```python
from build123d import *

# Parameters (mm, degrees)
SKETCH1_W                    = 76.2
SKETCH1_H                    = 127
BOSS_EXTRUDE1_DEPTH          = 24.13
SKETCH2_R                    = 7.9375
F_1_2_13_THREADED_HOLE_DEPTH = 78.885280381
SKETCH3_R                    = 5.0419
F_3_8_THROUGH_HOLES_DEPTH    = 78.885280381
SKETCH4_R                    = 21.43125
CUT_EXTRUDE1_DEPTH           = 9.525


with BuildPart() as part:
    # Sketch1 → Boss-Extrude1 (new body)
    with BuildSketch(Plane(origin=(0, 0, 0), x_dir=(1, 0, 0), z_dir=(0, 1, 0))):
        Rectangle(SKETCH1_W, SKETCH1_H)
    extrude(amount=BOSS_EXTRUDE1_DEPTH)

    # Sketch2 → 1/2"-13 Threaded Hole (cut, through all)
    with BuildSketch(Plane(origin=(0, 24.13, 0), x_dir=(1, 0, 0), z_dir=(0, 1, 0))):
        with Locations(Location((0, 0, 0), (0, 0, 270))):
            Circle(SKETCH2_R)
    extrude(amount=-F_1_2_13_THREADED_HOLE_DEPTH, mode=Mode.SUBTRACT)

    # Sketch3 → 3/8" Through Holes (cut, through all)
    with BuildSketch(Plane(origin=(0, 24.13, 0), x_dir=(1, 0, 0), z_dir=(0, 1, 0))):
        with Locations(Location((-19.05, 44.45, 0), (0, 0, 270))):
            Circle(SKETCH3_R)
        with Locations(Location((19.05, 44.45, 0), (0, 0, 270))):
            Circle(SKETCH3_R)
        with Locations(Location((19.05, -44.45, 0), (0, 0, 270))):
            Circle(SKETCH3_R)
        with Locations(Location((-19.05, -44.45, 0), (0, 0, 270))):
            Circle(SKETCH3_R)
    extrude(amount=-F_3_8_THROUGH_HOLES_DEPTH, mode=Mode.SUBTRACT)

    # Sketch4 → Cut-Extrude1 (cut)
    with BuildSketch(Plane(origin=(0, 24.13, 0), x_dir=(1, 0, 0), z_dir=(0, 1, 0))):
        with Locations(Location((0, 0, 0), (0, 0, 270))):
            Circle(SKETCH4_R)
    extrude(amount=-CUT_EXTRUDE1_DEPTH, mode=Mode.SUBTRACT)


solid = part.part
```
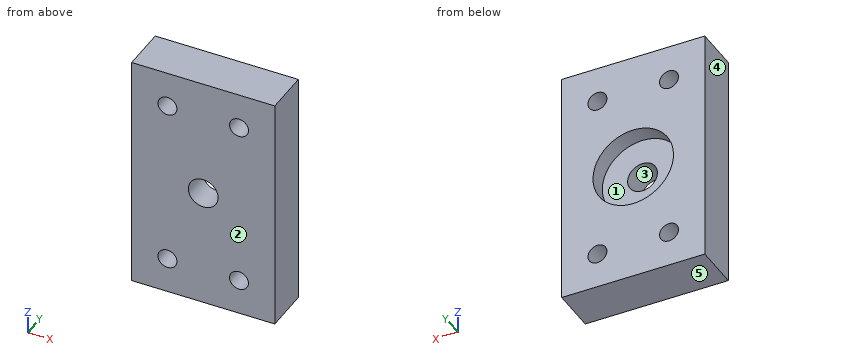
Here's how the part is built. I have some questions about the finished solid (model axes, mm). Face numbers are marked on the shaded views. A direction names the side the tool comes from. Coordinates: 2 decimals unless noted, no trailing zeros. Order: outer loops, then holes, each group sorted by start corner. A loop starts at its lowest first (then second) coordinate and runs counter-clockwise, first axis right, second up. Notation, with made-up numbers: (31.25, 47.25) - (38.25, 47.25) arc R30 cw to (38.25, 74.25) - close; hole circle Ø1 at (60.5, 59). An arc over 180 degrees is marked (long way). One line per question, with ' | ' between items.
(1) Suppose I cut it at A-A on z = -44.45. List the corners of the cut face in (x, y) for me.
Report:
outline: (-38.1, 0) - (-24.09, 0) - (-24.09, 24.13) - (-38.1, 24.13) - close; (-14.01, 0) - (14.01, 0) - (14.01, 24.13) - (-14.01, 24.13) - close; (24.09, 0) - (38.1, 0) - (38.1, 24.13) - (24.09, 24.13) - close
(2) Suppose I cut it at C-C on x = 0. List the corners of the cut face in (y, z) for me (1 decimal), and give its area (3 significant figures).
Report:
outline: (0, -63.5) - (24.1, -63.5) - (24.1, -21.4) - (14.6, -21.4) - (14.6, -7.9) - (0, -7.9) - close; (0, 7.9) - (14.6, 7.9) - (14.6, 21.4) - (24.1, 21.4) - (24.1, 63.5) - (0, 63.5) - close | area: 2,420 mm2
(3) Will these pins go through, and if not, where does the flat tip stop? pin 1 (16 mm diameter, centred on x = 19.05, z = 44.45, fed in from +Y); pin 2 (8 mm diameter, centred on x = -5.5, z = 9, fed in from +Y) (3 decimals); pin 3 (14.5 mm diameter, centred on x = 0, z = 0, fed in from -Y).
Report:
pin 1: stops at y = 24.13 | pin 2: stops at y = 14.605 | pin 3: passes through
(4) Suppose I cut it at B-B on z = 0. List the corners of the cut face in (x, y) for me (1 decimal), and give its area (3 significant figures).
Report:
outline: (-38.1, 0) - (-7.9, 0) - (-7.9, 14.6) - (-21.4, 14.6) - (-21.4, 24.1) - (-38.1, 24.1) - close; (7.9, 0) - (38.1, 0) - (38.1, 24.1) - (21.4, 24.1) - (21.4, 14.6) - (7.9, 14.6) - close | area: 1,200 mm2
(5) For the marked faces 1 and 2, which set-ups out of +Z, -Z, +X, -X, +Y, -Y let a thin tool reach every point of the face, with its end or its side?
Report:
face 1: +Y | face 2: +Z, -Z, +X, -X, -Y
(6) If we mould it in two halves opening along X, with no side actions, what happens to the marked faces 3, 4 and 5? For each: pulls with the +X half, pulls with the -X half, needs draft (parallel to the pull), parting line crosses it, or undercut.
Report:
face 3: undercut | face 4: pulls with the -X half | face 5: needs draft
(7) If I drill on L1, parallel to X at y = 9.5, z = -44; L2, parallel to Z at x = 17, y = 3; L3, parallel to Z at x = -21.5, y = 20, over which ranges is the centre line in solid material (lowest first)?
Report:
L1: x = -38.1 to -24.07, -14.03 to 14.03, 24.07 to 38.1 | L2: z = -63.5 to -49.06, -39.84 to 39.84, 49.06 to 63.5 | L3: z = -63.5 to -48.86, -40.04 to 40.04, 48.86 to 63.5
(8) Suppose I cut it at D-D on y = 10.5. State how many separate pieces and enclosed holes the cut face has, and give its area (3 significant figures).
Report:
separate pieces: 1 | enclosed holes: 5 | area: 9,160 mm2
